CAD build for the part. Positions are in the model's coordinates, mm. A direction names the side the tool comes from. Coordinates: 2 decimals unless noted, no trailing zeros. Loops run counter-clockwise (first coordinate to the right, second up) from the corner with the lowest first, then second, coordinate; pieces in that order, holes last. Notation, with made-up numbers: (1, -17.5) -> (5, -17.5) arc R25 ccw to (5, 15.5) -> close; hole circle Ø3 at (69, 63). An arc over 180 degrees is marked (long way). Answer as a JSON object with one key per item and string values. Group by question number.
Solid Edge part; units mm, degrees
sketch "Sketch1" plane through (0, 0, 15) normal (0, 0, 1) x (1, 0, 0)
  circle A0 centre (3.8798, 0.4153) radius 1.5
  circle A1 centre (33.5593, -102.2006) radius 1.5
  arc A2 (27.9428, 10.916) -> (42.9428, -4.084) centre (27.9428, -4.084) cw
  line L0 (42.9428, -4.084) -> (42.9428, -95.084)
  arc A3 (42.9428, -95.084) -> (27.9428, -110.084) centre (27.9428, -95.084) cw
  line L1 (27.9428, -110.084) -> (6.9428, -110.084)
  arc A4 (6.9428, -110.084) -> (-8.0572, -95.084) centre (6.9428, -95.084) cw
  line L2 (-8.0572, -95.084) -> (-8.0572, -4.084)
  arc A5 (-8.0572, -4.084) -> (6.9428, 10.916) centre (6.9428, -4.084) cw
  line L3 (6.9428, 10.916) -> (27.9428, 10.916)
  circle A6 centre (30.9691, 0.4033) radius 1.5
  circle A7 centre (1.1618, -101.9274) radius 1.5
extrude "Protrusion1" add sketch "Sketch1" along normal blind 2
sketch "Sketch2" plane through (17.4428, -49.584, 15) normal (0, 0, -1) x (0, -1, 0)
  arc A0 (-58.8, 10.5) -> (-45.5, 23.8) centre (-45.5, 10.5) cw
  line L0 (-45.5, 23.8) -> (45.5, 23.8)
  arc A1 (45.5, 23.8) -> (58.8, 10.5) centre (45.5, 10.5) cw
  line L1 (58.8, 10.5) -> (58.8, -10.5)
  arc A2 (58.8, -10.5) -> (45.5, -23.8) centre (45.5, -10.5) cw
  line L2 (45.5, -23.8) -> (-45.5, -23.8)
  arc A3 (-45.5, -23.8) -> (-58.8, -10.5) centre (-45.5, -10.5) cw
  line L3 (-58.8, -10.5) -> (-58.8, 10.5)
  arc A4 (-45.5, -22.3) -> (-57.3, -10.5) centre (-45.5, -10.5) cw
  line L4 (-57.3, -10.5) -> (-57.3, 10.5)
  arc A5 (-57.3, 10.5) -> (-45.5, 22.3) centre (-45.5, 10.5) cw
  line L5 (-45.5, 22.3) -> (45.5, 22.3)
  arc A6 (45.5, 22.3) -> (57.3, 10.5) centre (45.5, 10.5) cw
  line L6 (57.3, 10.5) -> (57.3, -10.5)
  arc A7 (57.3, -10.5) -> (45.5, -22.3) centre (45.5, -10.5) cw
  line L7 (45.5, -22.3) -> (-45.5, -22.3)
extrude "ExtrudedProtrusion_2" add sketch "Sketch2" along normal blind 3
sketch "Sketch3" plane through (17.4428, -108.384, 13.5) normal (0, -1, 0) x (-1, 0, 0)
  line L0 (-2, 1.5) -> (-2, 0.5)
  arc A0 (-2, 0.5) -> (2, 0.5) centre (0, 0.5) ccw
  line L1 (2, 0.5) -> (2, 1.5)
  line L2 (2, 1.5) -> (-2, 1.5)
extrude "ExtrudedCutout_1" cut sketch "Sketch3" against normal blind 2
Item 1: Band-saw the part on B-B, the plane x = 8.5. List the corners of the cut face in (y, z).
Item 2: Pull direction Y, two halves, no side cores. Call faces 4 (the cylindrical face through (-2.36, 5.42, 13.52)), 5 (the cylindrical face through (32.4, -0.05, 15.99)), 6 (the cylindrical face through (-2.565, -104.385, 13.521)): +Y half, -Y half, draft (parallel to the pull), parting line (faces both ways), or undercut.
Item 3: Drill centre lines: L1, parallel to X at y = -69, z = 12.35; L2, parallel to Y at x = 22.5, z = 13.4; L3, parallel to Z at x = 31, y = -70.5. Where is each one in solid material? Low to high.
Item 4: Band-saw the part on A-A, the plane y = -55. List the corners of the cut face in (x, z).
Item 5: 3-axis set-ups, long thin cutter, end or side, ignore diameter. For faces 1 (the cylindrical face through (36.378, 4.168, 13.521)), 2 (the flat face through (11, -108.384, 14)), 3 (the flat face through (-6.357, -49, 14)): which of +Z, -Z, +X, -X, +Y, -Y reach the whole face in a straight line?
Item 6: Flat gauge pins, fed straight in: P1, Ø0.9, axis at y = -45, z = 13, coming from the +X side; P2, Ø1.5, axis at x = 1, y = -19, coming from the -Z side; P3, Ø2.5, axis at y = -37, z = 13.5, coming from the -X side; P4, Ø2.5, axis at x = 33.56, y = -102.2, coming from the +Z side. Where does each tip first touch, or does it go through?
Reply:
{
 "1": {"outline": "(-110.08, 15) -> (-108.38, 15) -> (-108.38, 12) -> (-106.88, 12) -> (-106.88, 15) -> (7.72, 15) -> (7.72, 12) -> (9.22, 12) -> (9.22, 15) -> (10.92, 15) -> (10.92, 17) -> (-110.08, 17) -> close"},
 "2": {"face 4": "+Y half", "face 5": "undercut", "face 6": "-Y half"},
 "3": {"L1": "-6.36 to -4.86, 39.74 to 41.24", "L2": "-108.38 to -106.88, 7.72 to 9.22", "L3": "15 to 17"},
 "4": {"outline": "(-8.06, 15) -> (-6.36, 15) -> (-6.36, 12) -> (-4.86, 12) -> (-4.86, 15) -> (39.74, 15) -> (39.74, 12) -> (41.24, 12) -> (41.24, 15) -> (42.94, 15) -> (42.94, 17) -> (-8.06, 17) -> close"},
 "5": {"face 1": "-Z", "face 2": "-Z, +X, -X, -Y", "face 3": "-Z, -X, +Y, -Y"},
 "6": {"P1": "x = 41.24", "P2": "z = 15", "P3": "x = -6.36", "P4": "through"}
}
